from build123d import *

# Parameters (mm, degrees)
BOSS_EXTRUDE2_DEPTH = 62.5
SKETCH4_R           = 7.5
SKETCH4_W           = 6
SKETCH4_H           = 18
CUT_EXTRUDE1_DEPTH  = 125
FILLET1_R           = 5


with BuildPart() as part:
    # Sketch3 → Boss-Extrude2 (new body, symmetric)
    with BuildSketch(Plane(origin=(0, 0, 0), x_dir=(0, 0, -1), z_dir=(1, 0, 0))):
        with BuildLine():
            Line((-21.5, 213.548888359), (-21.5, 158.548888359))
            ThreePointArc((-21.5, 158.548888359), (0, 160), (21.5, 158.548888359))
            Line((21.5, 158.548888359), (21.5, 213.548888359))
            Line((21.5, 213.548888359), (13.5, 213.548888359))
            Line((13.5, 213.548888359), (13.5, 170))
            Line((13.5, 170), (-13.5, 170))
            Line((-13.5, 170), (-13.5, 213.548888359))
            Line((-13.5, 213.548888359), (-21.5, 213.548888359))
        make_face()
    extrude(amount=BOSS_EXTRUDE2_DEPTH, both=True)

    # Sketch4 → Cut-Extrude1 (cut)
    with BuildSketch(Plane.XY.offset(21.5)):
        with BuildLine():
            Line((62.5, 213.548888359), (-28.5, 213.548888359))
            ThreePointArc((-28.5, 213.548888359), (-25.924800571, 213.326179989), (-23.426070272, 212.66466808))
            Line((-23.426070272, 212.66466808), (62.5, 181.778464764))
            Line((62.5, 181.778464764), (62.5, 213.548888359))
        make_face()
        with BuildLine():
            ThreePointArc((-62.5, 183.691023983), (-62.119397663, 185.604441145), (-61.035533906, 187.226557889))
            Line((-61.035533906, 187.226557889), (-39.106601718, 209.155490077))
            ThreePointArc((-39.106601718, 209.155490077), (-34.240251485, 212.407081347), (-28.5, 213.548888359))
            Line((-28.5, 213.548888359), (-62.5, 213.548888359))
            Line((-62.5, 213.548888359), (-62.5, 183.691023983))
        make_face()
        Polygon((-56.5, 176.548888359), (-62.5, 176.548888359), (-62.5, 173.092612301), (-62.5, 158.548888359), (-56.5, 158.548888359), align=None)
        with Locations((-28.5, 198.548888359)):
            Circle(SKETCH4_R)
        with Locations((59.5, 167.548888359)):
            Rectangle(SKETCH4_W, SKETCH4_H)
    extrude(amount=-CUT_EXTRUDE1_DEPTH, mode=Mode.SUBTRACT)

    # Fillet1
    fillet1_edges = [part.edges().sort_by_distance(p)[0] for p in [
        (62.5, 181.778464764, 17.5),
        (62.5, 181.778464764, -17.5),
    ]]
    fillet(fillet1_edges, radius=FILLET1_R)


solid = part.part
Can you work these out from the model? Positions are in its coordinate system, mm. A direction names the side the tool comes from. Give positions to 0.01 mm unless a question says otherwise; leave off trailing zeros. Loops run counter-clockwise (first coordinate to the right, second up) from the corner with the lowest first, then second, coordinate; pieces in that order, holes last. Notation, with made-up numbers: (89.25, 78) -> (130.25, 78) arc R19 ccw to (130.25, 108) -> close; hole circle Ø3 at (2, -20.5). An arc over 180 degrees is marked (long way). Return JSON: item names as keys, results as strings.
Q1. I want a section at C-C, the plane x = 33.5. List the corners of the cut face in (y, z) for me.
Checks:
{"outline": "(158.55, -21.5) -> (192.2, -21.5) -> (192.2, -13.5) -> (170, -13.5) -> (170, 13.5) -> (192.2, 13.5) -> (192.2, 21.5) -> (158.55, 21.5) arc R160 cw to start"}
Q2. On a 3-axis mill with a long thin cutter (end or side, diameter ignored), from which of +Z, -Z, +X, -X, +Y, -Y can I reach the whole of each face in a straight line? I mean faces 1 (the face through (59, 176.549, -17)), 2 (the face through (-56.5, 167, 0)), 3 (the face through (1, 187, 13.5)). Say none if no direction works.
Checks:
{"face 1": "+Z, -Z, +X, -Y", "face 2": "+Z, -Z, -X, -Y", "face 3": "+X, -X, +Y"}
Q3. I want a section at B-B, the plane y = 185. List the corners of the cut face in (x, z) for me.
Checks:
{"outline": "(-62.33, -21.5) -> (53.54, -21.5) -> (53.54, -13.5) -> (-62.33, -13.5) -> close; (-62.33, 13.5) -> (53.54, 13.5) -> (53.54, 21.5) -> (-62.33, 21.5) -> close"}
Q4. For pin 1 Ø21.5 at (x, z) = (25, 0) entering from +Y; pin 2 Ø1.5 at (x, z) = (-17, 10) entering from -Y; pin 3 Ø1.8 at (x, z) = (59, 16) entering from -Y, each with a flat end and sliding along its axis, tell me the tip position at first contact or that it passes through.
Checks:
{"pin 1": "stops at y = 170", "pin 2": "stops at y = 159.64", "pin 3": "stops at y = 176.55"}
Q5. I want a section at A-A, the plane y = 203. List the corners of the cut face in (x, z) for me.
Checks:
{"outline": "(-45.26, -21.5) -> (-34.54, -21.5) -> (-34.54, -13.5) -> (-45.26, -13.5) -> close; (-45.26, 13.5) -> (-34.54, 13.5) -> (-34.54, 21.5) -> (-45.26, 21.5) -> close; (-22.46, -21.5) -> (3.46, -21.5) -> (3.46, -13.5) -> (-22.46, -13.5) -> close; (-22.46, 13.5) -> (3.46, 13.5) -> (3.46, 21.5) -> (-22.46, 21.5) -> close"}
Q6. I need wall thicknesses on probe 1 along Z at (x, y) = (22, 192); probe 2 along Y at (x, z) = (-28, 16); probe 3 along Y at (x, z) = (-28.5, -16.25). Which ranges of each line are inside material? Lowest first, please.
Checks:
{"probe 1": "z = -21.5 to -13.5, 13.5 to 21.5", "probe 2": "y = 159.2 to 191.07, 206.03 to 213.54", "probe 3": "y = 159.17 to 191.05, 206.05 to 213.55"}
Q7. I want a section at D-D, the plane z = -11. List the corners of the cut face in (x, y) for me, then the cut area to 3 significant figures.
Checks:
{"outline": "(-56.5, 159.62) -> (56.5, 159.62) -> (56.5, 170) -> (-56.5, 170) -> close", "area": "1,170 mm2"}
Q8. We'd pull the mould along Z, two halves only. Please class faces 4 (the face through (1, 180, 21.5)), 5 (the face through (-59, 176.549, -17)), 6 (the face through (1, 180, -21.5)), 7 (the face through (1, 160, 0)): released by +Z, released by -Z, zero draft, split by the parting line, or undercut.
Checks:
{"face 4": "released by +Z", "face 5": "zero draft", "face 6": "released by -Z", "face 7": "undercut"}
